```python
from build123d import *

# Parameters (mm, degrees)
BOSS_EXTRUDE1_DEPTH = 80


with BuildPart() as part:
    # Sketch1 → Boss-Extrude1 (new, symmetric)
    with BuildSketch(Plane(origin=(0, 0, 0), x_dir=(0, 0, -1), z_dir=(1, 0, 0))):
        with BuildLine():
            Line((0, -15.405), (0, 15.405))
            Line((0, 15.405), (-4.3, 15.405))
            Line((-4.3, 15.405), (-4.3, 13.955))
            Line((-4.3, 13.955), (-19.295662505, 12.238340714))
            ThreePointArc((-19.295662505, 12.238340714), (-32.08, 0), (-19.295662505, -12.238340714))
            Line((-19.295662505, -12.238340714), (-4.3, -13.955))
            Line((-4.3, -13.955), (-4.3, -15.405))
            Line((-4.3, -15.405), (0, -15.405))
        make_face()
    extrude(amount=BOSS_EXTRUDE1_DEPTH, both=True)


solid = part.part
```
Input: part model. Units: mm. Frame: model coordinates. Round coordinates to 2 decimals unless told otherwise and drop trailing zeros. Loops run counter-clockwise (first coordinate to the right, second up) from the corner with the lowest first, then second, coordinate; pieces in that order, holes last.
1) Pin query (flat end, axial travel): pin 1 (12 mm diameter, centred on x = -31, z = 7, fed in from -Y) (3 decimals); pin 2 (12 mm diameter, centred on x = 60, y = -8.5, fed in from +Z); pin 3 (1.2 mm diameter, centred on x = -10.5, y = -15, fed in from +Z); pin 4 (12 mm diameter, centred on x = -0.5, y = 10, fed in from +Z). Return the tip coordinate at first contact, or that it passes through.
Ans:
pin 1: stops at y = -15.405
pin 2: stops at z = 31.82
pin 3: stops at z = 4.3
pin 4: stops at z = 31.41
2) Section query A-A on x = 51. Return the cut outline in (y, z) (3 decimals), plus the area to 3 significant figures.
Ans:
outline: (-15.405, 0) - (15.405, 0) - (15.405, 4.3) - (13.955, 4.3) - (12.238, 19.296) arc R12.25 ccw (long way) to (-12.238, 19.296) - (-13.955, 4.3) - (-15.405, 4.3) - close
area: 774 mm2
3) Section query C-C on y = -8. Return the cut outline in (x, z), plus the area to 3 significant figures.
Ans:
outline: (-80, 0) - (80, 0) - (80, 29.11) - (-80, 29.11) - close
area: 4,660 mm2
4) Material intervals for line 1 (Y direction, x = -21, z = 20.5); line 2 (Y direction, x = -19.5, z = 28); line 3 (Z direction, x = 39.5, y = 10), sorted ascending.
Ans:
line 1: y = -12.23 to 12.23
line 2: y = -9.13 to 9.13
line 3: z = 0 to 26.91
5) Section query B-B on z = 26. Return the cut outline in (x, y), plus the area to 3 significant figures.
Ans:
outline: (-80, -10.58) - (80, -10.58) - (80, 10.58) - (-80, 10.58) - close
area: 3,390 mm2
